For this review, use the dimensioned drawing (mm, ordinates from the lowest corner) and the shaded views. A direction names the side the tool comes from. Coordinates: 2 decimals unless noted, no trailing zeros. Loops run counter-clockwise (first coordinate to the right, second up) from the corner with the lowest first, then second, coordinate; pieces in that order, holes last. Notation, with made-up numbers: M 69,25.5 L 123,25.5 A22 ccw 123,39.5 Z; hole C 13,79 d1. An arc over 180 degrees is marked long. One line per item, written item: value.
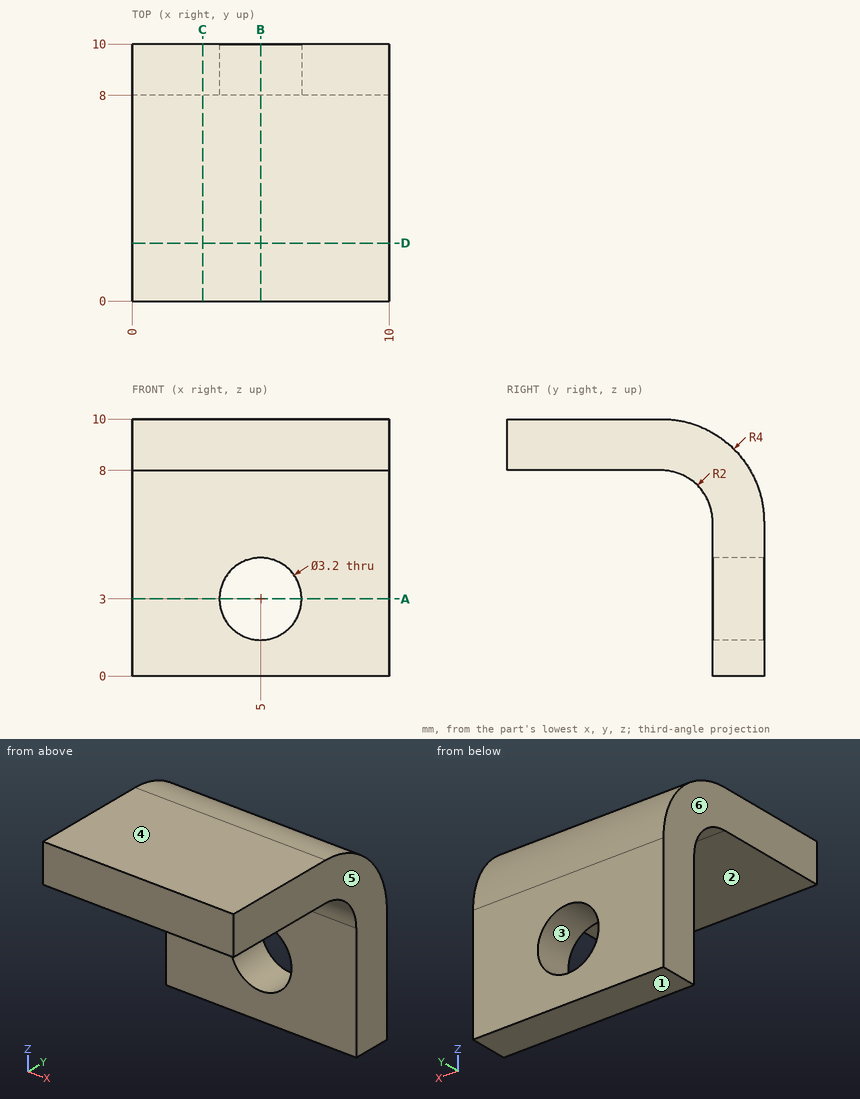
(1) We need section B-B on x = 5. State the section outline as (y, z) points.
Reply:
outline: M 0,8 L 6,8 A2 cw 8,6 L 8,4.6 L 10,4.6 L 10,6 A4 ccw 6,10 L 0,10 Z; M 8,0 L 10,0 L 10,1.4 L 8,1.4 Z
(2) Tool access review of the marked faces 1 and 2: name each direction out of +Z, -Z, +X, -X, +Y, -Y from which nothing blocks a thin tool from reaching the whole face with its end or side.
Reply:
face 1: -Z, +X, -X, +Y, -Y
face 2: -Z, +X, -X, -Y
(3) We need section C-C on x = 2.75. State the section outline as (y, z) points, then the cut area to 3 significant figures.
Reply:
outline: M 0,8 L 6,8 A2 cw 8,6 L 8,0 L 10,0 L 10,6 A4 ccw 6,10 L 0,10 Z
area: 33.4 mm2
(4) We need section D-D on y = 2.25. State the section outline as (x, z) points, then the cut area to 3 significant figures.
Reply:
outline: M 0,8 L 10,8 L 10,10 L 0,10 Z
area: 20.0 mm2
(5) Insertion check: pin 1 (4 mm diameter, centred on x = 2, y = 4, fed in from -Z); pin 2 (5 mm diameter, centred on x = 6.5, y = 4.5, fed in from -Z); pin 3 (4 mm diameter, centred on x = 5, z = 3, fed in from +Y); pin 4 (3 mm diameter, centred on x = 7, z = 8.5, fed in from +Y). Each pin has a flat end and moves straight along its axis. Give the tip position at first contact, or say it passes through.
Reply:
pin 1: stops at z = 8
pin 2: stops at z = 7.73
pin 3: stops at y = 10
pin 4: stops at y = 9.87
(6) We need section A-A on z = 3. State the section outline as (x, y) points, then the cut area to 3 significant figures.
Reply:
outline: M 0,8 L 3.4,8 L 3.4,10 L 0,10 Z; M 6.6,8 L 10,8 L 10,10 L 6.6,10 Z
area: 13.6 mm2
(7) Mouldability with a two-part tool opening along X and no side actions: class the marked faces 3, 4, 5 and 6 as released by +X, released by -X, zero draft, split by the parting line, or undercut.
Reply:
face 3: undercut
face 4: zero draft
face 5: released by +X
face 6: released by -X
(8) To check wall thickness, follow line 1 along X through (y, z) = (9.1, 3); line 2 along Y through (x, z) = (1.25, 3.25). State the ranges of each line that lie inside material, in increasing order. Write a range as [from, to].
Reply:
line 1: x = [0, 3.4], [6.6, 10]
line 2: y = [8, 10]
